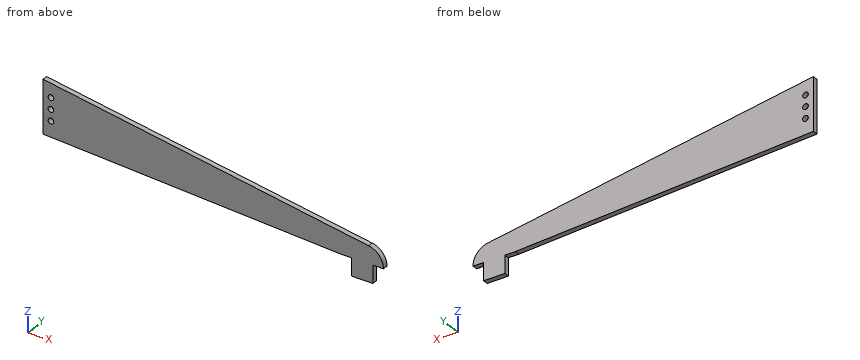
Autodesk Inventor part; units mm, degrees
ref_plane "YZ Plane" through (0, 0, 0) normal (1, 0, 0) x (0, 1, 0)
ref_plane "XZ Plane" through (0, 0, 0) normal (0, 1, 0) x (-1, 0, 0)
ref_plane "XY Plane" through (0, 0, 0) normal (0, 0, 1) x (1, 0, 0)
sketch "スケッチ3" plane through (0, 0, 0) normal (0, 1, 0) x (-1, 0, 0)
  line L0 (0, -35.3598) -> (0, -5.3598)
  line L1 (-187, -44.8598) -> (-187, -54.8598)
  line L2 (-175, -44.8598) -> (-175, -54.8598)
  line L3 (0, -5.3598) -> (-184.5847, -34.9862)
  arc A0 (-184.5847, -34.9862) -> (-193, -44.8598) centre (-183, -44.8598) ccw
  line L4 (-187, -54.8598) -> (-175, -54.8598)
  line L5 (-187, -44.8598) -> (-193, -44.8598)
  line L6 (0, -35.3598) -> (-169, -44.8598)
  line L7 (-169, -44.8598) -> (-175, -44.8598)
  circle A1 centre (-4.5, -20.3598) radius 1.6
  circle A2 centre (-4.5, -13.9598) radius 1.6
  circle A3 centre (-4.5, -26.7598) radius 1.6
  point P0 (0, -20.3598)
  dimension "d17" = 10
  dimension "d18" = 6
  dimension "d20" = 30
  dimension "d21" = 4.5
  dimension "d22" = 6.4
  dimension "d23" = 6.4
extrude "押し出し2" add sketch "スケッチ3" along normal blind 3
equation "\"d23\" = d22"
properties part number "SqPipe92" material "アクリル、クリア"
Can you work these out from the model? Positions are in its coordinate system, mm. Give positions to 0.01 mm unless a question says otherwise; leave off trailing zeros. Loops run counter-clockwise (first coordinate to the right, second up) from the corner with the lowest first, then second, coordinate; pieces in that order, holes last. Notation, with made-up numbers: (-10, -38.75) - (6, -38.75) arc R6 ccw to (6, -30.75) - close; hole circle Ø11 at (-39, 33). An arc over 180 degrees is marked (long way). Return JSON: item names as keys, results as strings.
1. I want a section at D-D on x = 27. Please give me the cut outline in (y, z).
Output values:
{"outline": "(0, -36.88) - (3, -36.88) - (3, -9.69) - (0, -9.69) - close"}
2. I want a section at A-A on x = 4.5. Please give me the cut outline in (y, z), and give its area (3 significant figures).
Output values:
{"outline": "(0, -35.61) - (3, -35.61) - (3, -28.36) - (0, -28.36) - close; (0, -25.16) - (3, -25.16) - (3, -21.96) - (0, -21.96) - close; (0, -18.76) - (3, -18.76) - (3, -15.56) - (0, -15.56) - close; (0, -12.36) - (3, -12.36) - (3, -6.08) - (0, -6.08) - close", "area": "59.8 mm²"}
3. I want a section at C-C on z = -39.5. Please give me the cut outline in (x, y), and give its area (3 significant figures).
Output values:
{"outline": "(73.65, 0) - (191.44, 0) - (191.44, 3) - (73.65, 3) - close", "area": "353 mm²"}
4. I want a section at B-B on y = 1.7. Please give me the cut outline in (x, z).
Output values:
{"outline": "(0, -35.36) - (169, -44.86) - (175, -44.86) - (175, -54.86) - (187, -54.86) - (187, -44.86) - (193, -44.86) arc R10 ccw to (184.58, -34.99) - (0, -5.36) - close; hole circle Ø3.2 at (4.5, -26.76); hole circle Ø3.2 at (4.5, -20.36); hole circle Ø3.2 at (4.5, -13.96)"}
5. If I drill on line 1 (Z direction, x = 4.5, y = 0.65); line 2 (Z direction, x = 103, y = 2.45); line 3 (Z direction, x = 112, y = 1.6), over which ranges is the centre line in solid material (lowest first)?
Output values:
{"line 1": "z = -35.61 to -28.36, -25.16 to -21.96, -18.76 to -15.56, -12.36 to -6.08", "line 2": "z = -41.15 to -21.89", "line 3": "z = -41.66 to -23.34"}
6. I'm going to push flat-ended pins straight in: pin 1 Ø1 at (x, y) = (65, 1.5) entering from +Z; pin 2 Ø3 at (x, z) = (78.5, -18) entering from -Y; pin 3 Ø1.9 at (x, z) = (4.5, -26.76) entering from -Y; pin 4 Ø1.5 at (y, z) = (2, -49.5) entering from -X. Where does each tip first touch, or does it pass through?
Output values:
{"pin 1": "stops at z = -15.71", "pin 2": "stops at y = 0", "pin 3": "passes through", "pin 4": "stops at x = 175"}
